from build123d import *

# Parameters (mm, degrees)
SKETCH_1_W          = 94
SKETCH_1_H          = 26
SKETCH_1_R          = 1
EXTRUDE_1_DEPTH     = 0.8
SKETCH_2_W          = 5.5
SKETCH_2_H          = 7.8
EXTRUDE_2_DEPTH     = 1
SKETCH_2_3_W        = 77.3
SKETCH_2_3_H        = 20.8
EXTRUDE_3_DEPTH     = 19.2
SKETCH_3_W          = 15.4
SKETCH_3_H          = 15.1
EXTRUDE_4_DEPTH     = 1.9
SKETCH_3_3_W        = 6.7
SKETCH_3_3_H        = 6.2
EXTRUDE_5_DEPTH     = 1
SKETCH_3_4_W        = 8.4
SKETCH_3_4_H        = 5.9
EXTRUDE_6_DEPTH     = 1.5
SKETCH_3_5_W        = 7.6
SKETCH_3_5_H        = 5.9
EXTRUDE_7_DEPTH     = 2.5
SKETCH_3_6_W        = 4.5
SKETCH_3_6_H        = 8.7
CUT_EXTRUDE_1_DEPTH = 53.706735812


with BuildPart() as part:
    # Sketch 1 → Extrude 1 (new body)
    with BuildSketch(Plane(origin=(0, 0, 0), x_dir=(1, 0, 0), z_dir=(0, 1, 0))):
        Rectangle(SKETCH_1_W, SKETCH_1_H)
        with Locations(Location((-44, 10, 0), (0, 0, 270))):
            Circle(SKETCH_1_R, mode=Mode.SUBTRACT)
        with Locations(Location((-44, -10, 0), (0, 0, 270))):
            Circle(SKETCH_1_R, mode=Mode.SUBTRACT)
        with Locations(Location((44, 10, 0), (0, 0, 270))):
            Circle(SKETCH_1_R, mode=Mode.SUBTRACT)
        with Locations(Location((44, -10, 0), (0, 0, 270))):
            Circle(SKETCH_1_R, mode=Mode.SUBTRACT)
    extrude(amount=EXTRUDE_1_DEPTH)

    # Sketch 2 → Extrude 2 (add)
    with BuildSketch(Plane(origin=(0, 0.8, 0), x_dir=(1, 0, 0), z_dir=(0, 1, 0))):
        with Locations((-39.45, 0)):
            Rectangle(SKETCH_2_W, SKETCH_2_H)
        with Locations((43.35, 0)):
            Rectangle(SKETCH_2_W, SKETCH_2_H)
    extrude(amount=EXTRUDE_2_DEPTH)

    # Sketch 2_3 → Extrude 3 (add)
    with BuildSketch(Plane(origin=(0, 0.8, 0), x_dir=(1, 0, 0), z_dir=(0, 1, 0))):
        with Locations((1.95, 0)):
            Rectangle(SKETCH_2_3_W, SKETCH_2_3_H)
    extrude(amount=EXTRUDE_3_DEPTH)

    # Sketch 3 → Extrude 4 (add)
    with BuildSketch(Plane.XZ):
        with Locations((32.9, 5.45)):
            Rectangle(SKETCH_3_W, SKETCH_3_H)
    extrude(amount=EXTRUDE_4_DEPTH)

    # Sketch 3_3 → Extrude 5 (add)
    with BuildSketch(Plane.XZ):
        with Locations((-27.35, 0)):
            Rectangle(SKETCH_3_3_W, SKETCH_3_3_H)
        with Locations((-16.075, 0)):
            Rectangle(SKETCH_3_3_W, SKETCH_3_3_H)
        with Locations((-4.8, 0)):
            Rectangle(SKETCH_3_3_W, SKETCH_3_3_H)
        with Locations((6.475, 0)):
            Rectangle(SKETCH_3_3_W, SKETCH_3_3_H)
        with Locations((17.75, 0)):
            Rectangle(SKETCH_3_3_W, SKETCH_3_3_H)
    extrude(amount=EXTRUDE_5_DEPTH)

    # Sketch 3_4 → Extrude 6 (add)
    with BuildSketch(Plane.XZ):
        with Locations((-27.5, 10.05)):
            Rectangle(SKETCH_3_4_W, SKETCH_3_4_H)
    extrude(amount=EXTRUDE_6_DEPTH)

    # Sketch 3_5 → Extrude 7 (add)
    with BuildSketch(Plane.XZ):
        with Locations((-37.2, 10.05)):
            Rectangle(SKETCH_3_5_W, SKETCH_3_5_H)
    extrude(amount=EXTRUDE_7_DEPTH)

    # Sketch 3_6 → Cut-Extrude 1 (cut, through all)
    with BuildSketch(Plane.XZ):
        with Locations((-44.75, 2.65)):
            Rectangle(SKETCH_3_6_W, SKETCH_3_6_H)
    extrude(amount=-CUT_EXTRUDE_1_DEPTH, mode=Mode.SUBTRACT)


solid = part.part
Check sheet for the modelled part. Datum: model origin and axes. Units: mm. A direction names the side the tool comes from. Give positions to 0.01 mm unless a question says otherwise; leave off trailing zeros. Loops run counter-clockwise (first coordinate to the right, second up) from the corner with the lowest first, then second, coordinate; pieces in that order, holes last. Notation, with made-up numbers: M 12,8.5 L 71,8.5 A36 cw 71,46.5 Z; hole C 26,-20.5 d5. An arc over 180 degrees is marked long. Return JSON: item names as keys, results as strings. Group by question number.
1. Mould release check, pull along Z, two halves, no side actions. Record for faces 5 (the flat face through (6, -1, 0)), 6 (the cylindrical face through (-43.01, 0.39, -10.13)), 7 (the flat face through (33, -1, -2.1)): released by +Z, released by -Z, zero draft, split by the parting line, or undercut.
2. Cross-section at B-B on x = -44. Record the boundary of the cut face in (y, z), plus the area to 3 significant figures.
3. Cross-section at C-C on z = -6.75. Record the boundary of the cut face in (x, y).
4. Cross-section at A-A on x = 44. Record the boundary of the cut face in (y, z).
5. Thickness scan on L1, parallel to X at y = 0.6, z = -10; L2, parallel to X at y = 15.5, z = 0; L3, parallel to Y at x = 27, z = 3.75. Record the ranges inside material, lowest first.
6. Go/stop test with flat-tipped pins: pin 1 (2 mm diameter, centred on y = -1.5, z = 10.5, fed in from +X); pin 2 (4 mm diameter, centred on x = 17, y = 7, fed in from -Z); pin 3 (0.5 mm diameter, centred on x = 6, y = -0.5, fed in from -Z). Record where each tip stops, or that it passes through.
7. Tool access check on faces 1 (the flat face through (-37, -1, 7.1)), 2 (the flat face through (33, -1.9, 6)), 3 (the flat face through (18, -1, 0)), 4 (the flat face through (-39, 1.8, 0)). Record the directions out of +Z, -Z, +X, -X, +Y, -Y that give a thin tool (end or side, any length) a straight path to the whole face; none if there is none.
8. Cross-section at D-D on y = 9. Record the boundary of the cut face in (x, z), plus the area to 3 significant figures.
Return value:
{
 "1": {"face 5": "zero draft", "face 6": "undercut", "face 7": "released by -Z"},
 "2": {"outline": "M 0,-13 L 0.8,-13 L 0.8,-11 L 0,-11 Z; M 0,-9 L 0.8,-9 L 0.8,-1.7 L 0,-1.7 Z; M 0,7 L 0.8,7 L 0.8,9 L 0,9 Z; M 0,11 L 0.8,11 L 0.8,13 L 0,13 Z", "area": "10.6 mm^2"},
 "3": {"outline": "M -47,0 L 47,0 L 47,0.8 L 40.6,0.8 L 40.6,20 L -36.7,20 L -36.7,0.8 L -47,0.8 Z"},
 "4": {"outline": "M 0,-13 L 0.8,-13 L 0.8,-11 L 0,-11 Z; M 0,-9 L 0.8,-9 L 0.8,-3.9 L 1.8,-3.9 L 1.8,3.9 L 0.8,3.9 L 0.8,9 L 0,9 Z; M 0,11 L 0.8,11 L 0.8,13 L 0,13 Z"},
 "5": {"L1": "-47 to -45, -43 to 43, 45 to 47", "L2": "-36.7 to 40.6", "L3": "-1.9 to 20"},
 "6": {"pin 1": "x = 40.6", "pin 2": "z = -10.4", "pin 3": "z = -3.1"},
 "7": {"face 1": "-Z, -X, -Y", "face 2": "+Z, -Z, +X, -Y", "face 3": "+Z, -Z, -X, -Y", "face 4": "+Z, -Z, -X, +Y"},
 "8": {"outline": "M -36.7,-10.4 L 40.6,-10.4 L 40.6,10.4 L -36.7,10.4 Z", "area": "1,610 mm^2"}
}
